Geometry: final body of the model. Coordinates: model frame, mm. A direction names the side the tool comes from. Give positions to 0.01 mm unless a question says otherwise; leave off trailing zeros. Order: outer loops, then holes, each group sorted by start corner. A loop starts at its lowest first (then second) coordinate and runs counter-clockwise, first axis right, second up. Notation, with made-up numbers: (48.5, -17) -> (80.5, -17) arc R11 cw to (80.5, 3) -> close; hole circle Ø4 at (60, -28.75). An arc over 180 degrees is marked (long way). Write item = value, one per line.
```python
from build123d import *

# Parameters (mm, degrees)
F0_W     = 20
F0_H     = 20
F0_R     = 2.5
F1_DEPTH = 5
F2_W     = 20
F2_H     = 5
F3_DEPTH = 20
F4_R     = 2.5
F5_DEPTH = 5.001
F6_R     = 5


with BuildPart() as f1:
    # F0 (on Top) → F1 (new body)
    with BuildSketch(Plane.XY):
        Rectangle(F0_W, F0_H)
        with Locations((0, 2)):
            Circle(F0_R, mode=Mode.SUBTRACT)
    extrude(amount=F1_DEPTH)

    # F2 (on face) → F3 (join)
    with BuildSketch(Plane.XY.offset(5)):
        with Locations((0, -7.5)):
            Rectangle(F2_W, F2_H)
    extrude(amount=F3_DEPTH)

    # F4 (on face) → F5 (cut, through all)
    with BuildSketch(Plane(origin=(0, -5, 0), x_dir=(-1, 0, 0), z_dir=(0, 1, 0))):
        with Locations((0, 17)):
            Circle(F4_R)
    extrude(amount=-F5_DEPTH, mode=Mode.SUBTRACT)

    # F6
    f6_edges = [f1.edges().sort_by_distance(p)[0] for p in [
        (-10, -7.5, 25),
        (10, -7.5, 25),
        (10, 10, 2.5),
        (-10, 10, 2.5),
    ]]
    fillet(f6_edges, radius=F6_R)


solid = f1.part
```
1) First-contact query: P1, Ø5, axis at x = 2, z = 13, coming from the +Y side; P2, Ø5, axis at x = 6, y = 4.5, coming from the +Z side. Flat tips, straight axial feed; report the tip coordinate or a pass-through.
Check sheet entries:
P1 = -5
P2 = 5
2) Section query B-B (z = 1.5). Output: boundary loops of the cut face in (x, y), plus the area to 3 significant figures.
Check sheet entries:
outline = (-10, -10) -> (10, -10) -> (10, 5) arc R5 ccw to (5, 10) -> (-5, 10) arc R5 ccw to (-10, 5) -> close; hole circle Ø5 at (0, 2)
area = 370 mm²
3) Mould query, pull axis Z, two halves, no side actions, for faces 1 (the face through (-1.34, -7.46, 19.11)), 2 (the face through (8, 9, 3)), 3 (the face through (0, -7, 25)). Classes: +Z half, -Z half, draft (parallel to the pull), parting line (faces both ways), or undercut.
Check sheet entries:
face_1 = undercut
face_2 = draft
face_3 = +Z half
4) Section query A-A (y = 2). Output: boundary loops of the cut face in (x, z).
Check sheet entries:
outline = (-10, 0) -> (-2.5, 0) -> (-2.5, 5) -> (-10, 5) -> close; (2.5, 0) -> (10, 0) -> (10, 5) -> (2.5, 5) -> close
5) Section query D-D (z = 17). Output: boundary loops of the cut face in (x, y), plus the area to 3 significant figures.
Check sheet entries:
outline = (-10, -10) -> (-2.5, -10) -> (-2.5, -5) -> (-10, -5) -> close; (2.5, -10) -> (10, -10) -> (10, -5) -> (2.5, -5) -> close
area = 75.0 mm²
6) Section query C-C (x = 0). Output: boundary loops of the cut face in (y, z).
Check sheet entries:
outline = (-10, 0) -> (-0.5, 0) -> (-0.5, 5) -> (-5, 5) -> (-5, 14.5) -> (-10, 14.5) -> close; (-10, 19.5) -> (-5, 19.5) -> (-5, 25) -> (-10, 25) -> close; (4.5, 0) -> (10, 0) -> (10, 5) -> (4.5, 5) -> close
7) Line query: line 1 (Z direction, x = 0, y = -7.2); line 2 (Y direction, x = 0, z = 2.1); line 3 (Z direction, x = -7, y = 1.5). Output: solid intervals per line, ascending. Write a range as from..to.
Check sheet entries:
line_1 = 0..14.5, 19.5..25
line_2 = -10..-0.5, 4.5..10
line_3 = 0..5
8) Reachability of faces 4 (the face through (8, -7, 24)), 5 (the face through (-2, 4, 5)) from +Z, -Z, +X, -X, +Y, -Y: full face, straight path, thin tool, end or side. Return the list, or none.
Check sheet entries:
face_4 = +Z, +X, +Y, -Y
face_5 = +Z, +X, -X, +Y
